Input: part model. Units: mm. Frame: model coordinates. A direction names the side the tool comes from. Give positions to 0.01 mm unless a question says otherwise; leave off trailing zeros. Write each loop counter-clockwise with the first axis right and the second up, starting at its lowest first coordinate (ties: lowest second). Pieces come first, ordered by that corner, then holes.
```python
from build123d import *

# Parameters (mm, degrees)
SKETCH1_R           = 1.5
SKETCH1_R_2         = 0.75
BOSS_EXTRUDE1_DEPTH = 2
SKETCH1_3_W         = 20
SKETCH1_3_H         = 10
BOSS_EXTRUDE2_DEPTH = 1
SKETCH1_4_R         = 0.75
CUT_EXTRUDE1_DEPTH  = 1
SKETCH1_5_W         = 20
SKETCH1_5_H         = 10
SKETCH1_5_W_2       = 18
SKETCH1_5_H_2       = 8
SKETCH1_5_R         = 2.035533906
SKETCH1_5_R_2       = 1.5
BOSS_EXTRUDE3_DEPTH = 1


with BuildPart() as part:
    # Sketch1 → Boss-Extrude1 (new body)
    with BuildSketch(Plane(origin=(0, 0, 0), x_dir=(1, 0, 0), z_dir=(0, 1, 0))):
        with Locations(Location((-7.5, 2.5, 0), (0, 0, 270))):
            Circle(SKETCH1_R)
        with Locations(Location((-2.5, 2.5, 0), (0, 0, 270))):
            Circle(SKETCH1_R)
        with Locations(Location((2.5, 2.5, 0), (0, 0, 270))):
            Circle(SKETCH1_R)
        with Locations(Location((7.5, 2.5, 0), (0, 0, 270))):
            Circle(SKETCH1_R)
        with Locations(Location((7.5, -2.5, 0), (0, 0, 270))):
            Circle(SKETCH1_R)
        with Locations(Location((2.5, -2.5, 0), (0, 0, 270))):
            Circle(SKETCH1_R)
        with Locations(Location((-2.5, -2.5, 0), (0, 0, 270))):
            Circle(SKETCH1_R)
        with Locations(Location((-7.5, -2.5, 0), (0, 0, 270))):
            Circle(SKETCH1_R)
        with Locations((-7.5, 2.5)):
            Circle(SKETCH1_R_2)
        with Locations((-2.5, 2.5)):
            Circle(SKETCH1_R_2)
        with Locations((2.5, 2.5)):
            Circle(SKETCH1_R_2)
        with Locations((7.5, 2.5)):
            Circle(SKETCH1_R_2)
        with Locations((7.5, -2.5)):
            Circle(SKETCH1_R_2)
        with Locations((2.5, -2.5)):
            Circle(SKETCH1_R_2)
        with Locations((-2.5, -2.5)):
            Circle(SKETCH1_R_2)
        with Locations((-7.5, -2.5)):
            Circle(SKETCH1_R_2)
    extrude(amount=BOSS_EXTRUDE1_DEPTH)

    # Sketch1_3 → Boss-Extrude2 (add)
    with BuildSketch(Plane(origin=(0, 0, 0), x_dir=(1, 0, 0), z_dir=(0, 1, 0))):
        Rectangle(SKETCH1_3_W, SKETCH1_3_H)
    extrude(amount=BOSS_EXTRUDE2_DEPTH)

    # Sketch1_4 → Cut-Extrude1 (cut)
    with BuildSketch(Plane(origin=(0, 0, 0), x_dir=(1, 0, 0), z_dir=(0, 1, 0))):
        with Locations(Location((-7.5, 2.5, 0), (0, 0, 270))):
            Circle(SKETCH1_4_R)
        with Locations(Location((-7.5, -2.5, 0), (0, 0, 270))):
            Circle(SKETCH1_4_R)
        with Locations(Location((-2.5, -2.5, 0), (0, 0, 270))):
            Circle(SKETCH1_4_R)
        with Locations(Location((-2.5, 2.5, 0), (0, 0, 270))):
            Circle(SKETCH1_4_R)
        with Locations(Location((2.5, -2.5, 0), (0, 0, 270))):
            Circle(SKETCH1_4_R)
        with Locations(Location((2.5, 2.5, 0), (0, 0, 270))):
            Circle(SKETCH1_4_R)
        with Locations(Location((7.5, -2.5, 0), (0, 0, 270))):
            Circle(SKETCH1_4_R)
        with Locations(Location((7.5, 2.5, 0), (0, 0, 270))):
            Circle(SKETCH1_4_R)
    extrude(amount=CUT_EXTRUDE1_DEPTH, mode=Mode.SUBTRACT)

    # Sketch1_5 → Boss-Extrude3 (add)
    with BuildSketch(Plane(origin=(0, 0, 0), x_dir=(1, 0, 0), z_dir=(0, 1, 0))):
        Rectangle(SKETCH1_5_W, SKETCH1_5_H)
        Rectangle(SKETCH1_5_W_2, SKETCH1_5_H_2, mode=Mode.SUBTRACT)
        with Locations(Location((5, 0, 0), (0, 0, 270))):
            Circle(SKETCH1_5_R)
        with Locations(Location((5, 0, 0), (0, 0, 270))):
            Circle(SKETCH1_5_R_2, mode=Mode.SUBTRACT)
        with Locations(Location((0, 0, 0), (0, 0, 270))):
            Circle(SKETCH1_5_R)
        with Locations(Location((0, 0, 0), (0, 0, 270))):
            Circle(SKETCH1_5_R_2, mode=Mode.SUBTRACT)
        with Locations(Location((-5, 0, 0), (0, 0, 270))):
            Circle(SKETCH1_5_R)
        with Locations(Location((-5, 0, 0), (0, 0, 270))):
            Circle(SKETCH1_5_R_2, mode=Mode.SUBTRACT)
    extrude(amount=-BOSS_EXTRUDE3_DEPTH)


solid = part.part
```
Item 1: Pin query (flat end, axial travel): pin 1 (0.9 mm diameter, centred on x = -7.5, z = -2.5, fed in from -Y); pin 2 (1 mm diameter, centred on x = 6, z = -2.5, fed in from -Y). Return the tip coordinate at first contact, or that it passes through.
Item 2: Set-up query: faces 5 (the cylindrical face through (-2.275, 0.493, 3.215)), 6 (the flat face through (10, 0, 0)), 7 (the cylindrical face through (1.036, 1.493, 2.175)). Return all of +Z, -Z, +X, -X, +Y, -Y with unobstructed straight access to the full face (end or side cutting, diameter ignored); none if empty.
Item 3: Section D-D (y = 0.2). Give the number of separate pieces and of enclosed holes in the cut face, and give its area (3 significant figures).
Item 4: Ray query, line 1 (X direction, y = 0.6, z = 2.5); line 2 (Z direction, x = 4.25, y = -0.35); line 3 (X direction, y = -0.15, z = -2.5). Return the intervals inside material, ascending.
Item 5: Section B-B (x = 0). Return loops of the section in (y, z).
Item 6: Mould query, pull axis Z, two halves, no side actions, for faces 1 (the flat face through (0, 0, 5)), 2 (the flat face through (-7.5, 1, -2.5)), 3 (the flat face through (0, 0, -5)), 4 (the flat face through (-2, 0, -1)). Classes: +Z half, -Z half, draft (parallel to the pull), parting line (faces both ways), or undercut.
Item 7: Section A-A (y = 1.3). Return loops of the section in (x, z), and give its area (3 significant figures).
Solved:
1. pin 1: stops at y = 1
1. pin 2: stops at y = 0
2. face 5: -Y
2. face 6: +Z, -Z, +X, +Y, -Y
2. face 7: +Y
3. separate pieces: 1
3. enclosed holes: 8
3. area: 186 mm2
4. line 1: x = -10 to -8.25, -6.75 to -3.25, -1.75 to 1.75, 3.25 to 6.75, 8.25 to 10
4. line 2: z = -5 to -4, -1.89 to -1.3, 1.3 to 1.89, 4 to 5
4. line 3: x = -10 to -9, 9 to 10
5. outline: (-1, -5) - (1, -5) - (1, 5) - (-1, 5) - (-1, 4) - (0, 4) - (0, 2.04) - (-1, 2.04) - (-1, 1.5) - (0, 1.5) - (0, -1.5) - (-1, -1.5) - (-1, -2.04) - (0, -2.04) - (0, -4) - (-1, -4) - close
6. face 1: +Z half
6. face 2: undercut
6. face 3: -Z half
6. face 4: undercut
7. outline: circle Ø3 at (-7.5, -2.5); circle Ø3 at (-7.5, 2.5); circle Ø3 at (-2.5, -2.5); circle Ø3 at (-2.5, 2.5); circle Ø3 at (2.5, -2.5); circle Ø3 at (2.5, 2.5); circle Ø3 at (7.5, -2.5); circle Ø3 at (7.5, 2.5)
7. area: 56.5 mm2
